```python
from build123d import *

# Parameters (mm, degrees)
CROQUIS1_W                 = 50
CROQUIS1_H                 = 25
SALIENTE_EXTRUIR1_DEPTH    = 10
CROQUIS2_W                 = 16.666666667
CROQUIS2_H                 = 25
SALIENTE_EXTRUIR2_DEPTH    = 20
CORTAR_EXTRUIR1_DEPTH      = 64.442887702
CORTAR_EXTRUIR1_DEPTH_BACK = 64.442887702
CROQUIS5_W                 = 5
CROQUIS5_H                 = 8.331666666
CORTAR_EXTRUIR3_DEPTH      = 47.368092477


with BuildPart() as part:
    # Croquis1 → Saliente-Extruir1 (new body)
    with BuildSketch(Plane(origin=(0, 0, 0), x_dir=(0, 0, -1), z_dir=(1, 0, 0))):
        with Locations((0, 12.5)):
            Rectangle(CROQUIS1_W, CROQUIS1_H)
    extrude(amount=SALIENTE_EXTRUIR1_DEPTH)

    # Croquis2 → Saliente-Extruir2 (add)
    with BuildSketch(Plane(origin=(10, 0, 0), x_dir=(0, 0, -1), z_dir=(1, 0, 0))):
        with Locations((-12.496666667, 12.5)):
            Rectangle(CROQUIS2_W, CROQUIS2_H)
        with Locations((12.501666667, 12.5)):
            Rectangle(CROQUIS2_W, CROQUIS2_H)
    extrude(amount=SALIENTE_EXTRUIR2_DEPTH)

    # Croquis3 → Cortar-Extruir1 (cut, two sides: drawn at the far end of the back side and taken through both)
    with BuildSketch(Plane.XY.offset(25).offset(-CORTAR_EXTRUIR1_DEPTH_BACK)):
        Polygon((-85.10047698, 47.802604082), (0, 25), (30, 16.961524227), (115.10047698, -5.841079855), (160.705685145, 164.359874105), (-39.495268815, 218.003558043), align=None)
    extrude(amount=CORTAR_EXTRUIR1_DEPTH + CORTAR_EXTRUIR1_DEPTH_BACK, mode=Mode.SUBTRACT)

    # Croquis5 → Cortar-Extruir3 (cut, through all)
    with BuildSketch(Plane.XZ):
        with Locations((7.5, -0.0025)):
            Rectangle(CROQUIS5_W, CROQUIS5_H)
    extrude(amount=-CORTAR_EXTRUIR3_DEPTH, mode=Mode.SUBTRACT)


solid = part.part
```
Work out the finished part from the listing and answer in its coordinate system (mm). A direction names the side the tool comes from. Round coordinates to 2 decimals unless told otherwise and drop trailing zeros. Loops run counter-clockwise (first coordinate to the right, second up) from the corner with the lowest first, then second, coordinate; pieces in that order, holes last. Notation, with made-up numbers: (58.25, 10) -> (85.25, 10) arc R11 ccw to (85.25, 29) -> close; hole circle Ø10 at (-35.5, 87.5). An arc over 180 degrees is marked (long way). Write each question's results on one line, items separated by ' | '. Start each with the question number.
1. Section D-D (z = -8) is taken. Determine the outline of the cut face in (x, y), plus the area to 3 significant figures.
2. Section B-B (y = 11) is taken. Determine the outline of the cut face in (x, z) (3 decimals).
3. Section A-A (x = 12.25) is taken. Determine the outline of the cut face in (y, z) (3 decimals), plus the area to 3 significant figures.
4. A tool of negligible diameter and unlimited length cuts with its end or side. For faces 1 (the face through (14.79, 21.037, -5.906)), 2 (the face through (20, 11, 20.83)), 3 (the face through (10, 11, -23)), 4 (the face through (17, 9, -4.168)), from which of +Z, -Z, +X, -X, +Y, -Y can it reach the whole face along a straight path? Write none if from no direction.
5. Find the intervals of material crossed by probe 1 along Z at (x, y) = (11.75, 5.75) (3 decimals); probe 2 along Z at (x, y) = (5.25, 18.25); probe 3 along X at (y, z) = (11.25, 23), in increasing order. Write a range as from..to.
6. For a pull along Z with two mould halves and no side action, classify faces 5 (the face through (0, 13, 0)), 6 (the face through (5, 12, 25)), 7 (the face through (5, 12, 0)) as +Z half, -Z half, draft (parallel to the pull), parting line (faces both ways), or undercut.
7. Section C-C (x = 15.25) is taken. Determine the outline of the cut face in (y, z) (3 decimals), plus the area to 3 significant figures.
8. Given pin 1 Ø4 at (y, z) = (22, -0.5) entering from +X; pin 2 Ø3 at (x, z) = (3.5, -13) entering from +Y; pin 3 Ø1.3 at (y, z) = (16, 23) entering from +X, each flat-ended and moving along its own axis, determine where each tip first touches the part or whether it passes through.
Evaluation:
1) outline: (0, 0) -> (30, 0) -> (30, 16.96) -> (0, 25) -> close | area: 629 mm2
2) outline: (0, -25) -> (10, -25) -> (10, -20.835) -> (30, -20.835) -> (30, -4.168) -> (5, -4.168) -> (5, 4.163) -> (30, 4.163) -> (30, 20.83) -> (10, 20.83) -> (10, 25) -> (0, 25) -> close
3) outline: (0, -20.835) -> (21.718, -20.835) -> (21.718, -4.168) -> (0, -4.168) -> close; (0, 4.163) -> (21.718, 4.163) -> (21.718, 20.83) -> (0, 20.83) -> close | area: 724 mm2
4) face 1: +Z, -Z, +X, +Y | face 2: +Z, +X, +Y, -Y | face 3: -Z, +X, +Y, -Y | face 4: +X, +Y, -Y
5) probe 1: z = -20.835..-4.168, 4.163..20.83 | probe 2: z = -25..-4.17, 4.16..25 | probe 3: x = 0..10
6) face 5: draft | face 6: +Z half | face 7: undercut
7) outline: (0, -20.835) -> (20.914, -20.835) -> (20.914, -4.168) -> (0, -4.168) -> close; (0, 4.163) -> (20.914, 4.163) -> (20.914, 20.83) -> (0, 20.83) -> close | area: 697 mm2
8) pin 1: stops at x = 5 | pin 2: stops at y = 24.46 | pin 3: stops at x = 10
